from build123d import *

# Parameters (mm, degrees)
F0_R          = 3
F0_R_2        = 2.5
F1_DEPTH      = 280.86
F2_R          = 2
F3_R          = 7
F6_DEPTH      = 30
F6_DEPTH_BACK = 30


# Not quite as in the source:
# - a feature names something its author has since deleted; it is built from what else it names


with BuildPart() as f1:
    # F0 (on Top) → F1 (new body)
    with BuildSketch(Plane.XY):
        with BuildLine():
            Line((18.15, -30), (30, -30))
            Line((30, -30), (30, -18.15))
            Line((30, -18.15), (27.5, -18.15))
            Line((27.5, -18.15), (27.5, -20.15))
            Line((27.5, -20.15), (21.5477069044, -20.15))
            ThreePointArc((21.5477069044, -20.15), (19.5, -15), (21.5477069044, -9.85))
            Line((21.5477069044, -9.85), (27.5, -9.85))
            Line((27.5, -9.85), (27.5, -11.85))
            Line((27.5, -11.85), (30, -11.85))
            Line((30, -11.85), (30, 11.85))
            Line((30, 11.85), (27.5, 11.85))
            Line((27.5, 11.85), (27.5, 9.85))
            Line((27.5, 9.85), (21.5477069044, 9.85))
            ThreePointArc((21.5477069044, 9.85), (19.5, 15), (21.5477069044, 20.15))
            Line((21.5477069044, 20.15), (27.5, 20.15))
            Line((27.5, 20.15), (27.5, 18.15))
            Line((27.5, 18.15), (30, 18.15))
            Line((30, 18.15), (30, 30))
            Line((30, 30), (18.15, 30))
            Line((18.15, 30), (18.15, 27.5))
            Line((18.15, 27.5), (20.15, 27.5))
            Line((20.15, 27.5), (20.15, 21.5477069044))
            ThreePointArc((20.15, 21.5477069044), (15, 19.5), (9.85, 21.5477069044))
            Line((9.85, 21.5477069044), (9.85, 27.5))
            Line((9.85, 27.5), (11.85, 27.5))
            Line((11.85, 27.5), (11.85, 30))
            Line((11.85, 30), (-11.85, 30))
            Line((-11.85, 30), (-11.85, 27.5))
            Line((-11.85, 27.5), (-9.85, 27.5))
            Line((-9.85, 27.5), (-9.85, 21.5477069044))
            ThreePointArc((-9.85, 21.5477069044), (-15, 19.5), (-20.15, 21.5477069044))
            Line((-20.15, 21.5477069044), (-20.15, 27.5))
            Line((-20.15, 27.5), (-18.15, 27.5))
            Line((-18.15, 27.5), (-18.15, 30))
            Line((-18.15, 30), (-30, 30))
            Line((-30, 30), (-30, 18.15))
            Line((-30, 18.15), (-27.5, 18.15))
            Line((-27.5, 18.15), (-27.5, 20.15))
            Line((-27.5, 20.15), (-21.5477069044, 20.15))
            ThreePointArc((-21.5477069044, 20.15), (-19.5, 15), (-21.5477069044, 9.85))
            Line((-21.5477069044, 9.85), (-27.5, 9.85))
            Line((-27.5, 9.85), (-27.5, 11.85))
            Line((-27.5, 11.85), (-30, 11.85))
            Line((-30, 11.85), (-30, -11.85))
            Line((-30, -11.85), (-27.5, -11.85))
            Line((-27.5, -11.85), (-27.5, -9.85))
            Line((-27.5, -9.85), (-21.5477069044, -9.85))
            ThreePointArc((-21.5477069044, -9.85), (-19.5, -15), (-21.5477069044, -20.15))
            Line((-21.5477069044, -20.15), (-27.5, -20.15))
            Line((-27.5, -20.15), (-27.5, -18.15))
            Line((-27.5, -18.15), (-30, -18.15))
            Line((-30, -18.15), (-30, -30))
            Line((-30, -30), (-18.15, -30))
            Line((-18.15, -30), (-18.15, -27.5))
            Line((-18.15, -27.5), (-20.15, -27.5))
            Line((-20.15, -27.5), (-20.15, -21.5477069044))
            ThreePointArc((-20.15, -21.5477069044), (-15, -19.5), (-9.85, -21.5477069044))
            Line((-9.85, -21.5477069044), (-9.85, -27.5))
            Line((-9.85, -27.5), (-11.85, -27.5))
            Line((-11.85, -27.5), (-11.85, -30))
            Line((-11.85, -30), (11.85, -30))
            Line((11.85, -30), (11.85, -27.5))
            Line((11.85, -27.5), (9.85, -27.5))
            Line((9.85, -27.5), (9.85, -21.5477069044))
            ThreePointArc((9.85, -21.5477069044), (15, -19.5), (20.15, -21.5477069044))
            Line((20.15, -21.5477069044), (20.15, -27.5))
            Line((20.15, -27.5), (18.15, -27.5))
            Line((18.15, -27.5), (18.15, -30))
        make_face()
        with Locations((-25, -25)):
            Circle(F0_R, mode=Mode.SUBTRACT)
        with Locations((-15, -15)):
            Circle(F0_R_2, mode=Mode.SUBTRACT)
        with Locations((25, -25)):
            Circle(F0_R, mode=Mode.SUBTRACT)
        with Locations((15, -15)):
            Circle(F0_R_2, mode=Mode.SUBTRACT)
        with Locations((-25, 25)):
            Circle(F0_R, mode=Mode.SUBTRACT)
        with Locations((-15, 15)):
            Circle(F0_R_2, mode=Mode.SUBTRACT)
        Polygon((-7, 22), (-7, 27.5), (0, 27.5), (7, 27.5), (7, 22), (10, 16), (10, 10), (16, 10), (22, 7), (27.5, 7), (27.5, 0), (27.5, -7), (22, -7), (16, -10), (10, -10), (10, -16), (7, -22), (7, -27.5), (0, -27.5), (-7, -27.5), (-7, -22), (-10, -16), (-10, -10), (-16, -10), (-22, -7), (-27.5, -7), (-27.5, 0), (-27.5, 7), (-22, 7), (-16, 10), (-10, 10), (-10, 16), align=None, mode=Mode.SUBTRACT)
        with Locations((15, 15)):
            Circle(F0_R_2, mode=Mode.SUBTRACT)
        with Locations((25, 25)):
            Circle(F0_R, mode=Mode.SUBTRACT)
    extrude(amount=F1_DEPTH)

    # F2
    f2_edges = [f1.edges().sort_by_distance(p)[0] for p in [
        (-7, 27.5, 140.43),
        (7, 27.5, 140.43),
    ]]
    fillet(f2_edges, radius=F2_R)

    # F3
    f3_edges = [f1.edges().sort_by_distance(p)[0] for p in [
        (-10, 16, 140.43),
        (10, 16, 140.43),
    ]]
    fillet(f3_edges, radius=F3_R)

    # F5 (on Right) → F6 (cut, two sides)
    with BuildSketch(Plane.YZ) as f6_sk:
        Polygon((166.5976946582, -66.7170951811), (146.3493769552, 35.0780720561), (-30, 0), (-9.751682297, -101.7951672372), align=None)
        Polygon((135.5963626007, 247.9208354856), (151.7094622056, 328.9268574701), (-13.8869003951, 361.8660219845), (-30, 280.86), align=None)
    extrude(amount=F6_DEPTH, mode=Mode.SUBTRACT)
    extrude(f6_sk.sketch, amount=-F6_DEPTH_BACK, mode=Mode.SUBTRACT)


solid = f1.part
Here's how the part is built. I have some questions about the finished solid (model axes, mm). Coordinates: 2 decimals unless noted, no trailing zeros. Order: outer loops, then holes, each group sorted by start corner. A loop starts at its lowest first (then second) coordinate and runs counter-clockwise, first axis right, second up. Notation, with made-up numbers: M -8,56.5 L 23,56.5 A20 ccw 23,85.5 Z; hole C 36.25,35.5 d3. An arc over 180 degrees is marked long. Answer as CSV lines item,"result". Start each with the question number.
1. For pin 1 (4 mm diameter, centred on x = 22, y = 23, fed in from +Z); pin 2 (1 mm diameter, centred on x = -16.5, z = 165, fed in from -Y); pin 3 (6 mm diameter, centred on x = 18.5, y = -6, fed in from -Z), each with a flat end and sliding along its axis, tell me the tip position at first contact or that it passes through.
2. We'd pull the mould along X, two halves only. Please class faces 1 (the flat face through (30, 0, 139)), 2 (the flat face through (-20.15, 24, 139)): released by +X, released by -X, zero draft, split by the parting line, or undercut.
3. I want a section at B-B, the plane x = 25. Write out the boundary of the cut face in (y, z).
4. I want a section at A-A, the plane y = -4. Write out the boundary of the cut face in (x, z), and give its area (3 significant figures).
5. I need wall thicknesses on line 1 (X direction, y = -15.5, z = 214.5); line 2 (X direction, y = 25, z = 124); line 3 (Y direction, x = -15, z = 131). Which ranges of each line are inside material? Lowest first, please. Write a range as [from, to].
6. I want a section at C-C, the plane z = 128.5. Count the separate pieces of the cut face and the enclosed holes in it, and give its area (3 significant figures).
Recorded:
1,pin 1,"stops at z = 270.72"
1,pin 2,"stops at y = -19.77"
1,pin 3,"stops at z = 4.18"
2,face 1,"released by +X"
2,face 2,"undercut"
3,outline,"M -30,0 L -28,0.4 L -28,280.46 L -30,280.86 Z; M -22,1.59 L -20.15,1.96 L -20.15,278.9 L -22,279.27 Z; M -9.85,4.01 L -7,4.57 L -7,276.29 L -9.85,276.85 Z; M 7,7.36 L 9.85,7.93 L 9.85,272.93 L 7,273.5 Z; M 20.15,9.98 L 22,10.34 L 22,270.52 L 20.15,270.88 Z; M 28,11.54 L 30,11.93 L 30,268.93 L 28,269.32 Z"
4,outline,"M -30,5.17 L -27.5,5.17 L -27.5,275.69 L -30,275.69 Z; M 27.5,5.17 L 30,5.17 L 30,275.69 L 27.5,275.69 Z"
4,area,"1,350 mm2"
5,line 1,"x = [-19.52, -17.45], [-12.55, -10], [10, 12.55], [17.45, 19.52]"
5,line 2,"x = [-30, -28], [-22, -20.15], [-9.85, -7], [7, 9.85], [20.15, 22], [28, 30]"
5,line 3,"y = [-19.5, -17.5], [-12.5, -10], [10, 12.5], [17.5, 19.5]"
6,separate pieces,"1"
6,enclosed holes,"9"
6,area,"1,080 mm2"
